```python
from build123d import *

# Parameters (mm, degrees)
F1_DEPTH = 25


with BuildPart() as f1:
    # F0 (on Right) → F1 (new body, symmetric)
    with BuildSketch(Plane.YZ):
        with BuildLine():
            Line((-68.631068, 16), (-68.631068, 0))
            Line((-68.631068, 0), (-44.032769, 0))
            Line((-44.032769, 0), (-44.032769, -22))
            Line((-44.032769, -22), (-25.631068, -22))
            ThreePointArc((-25.631068, -22), (-2.631068, 0.150878), (20.368932, -22))
            Line((20.368932, -22), (38.770634, -22))
            Line((38.770634, -22), (38.770634, 0))
            Line((38.770634, 0), (63.368932, 0))
            Line((63.368932, 0), (63.368932, 16))
            Line((63.368932, 16), (-68.631068, 16))
        make_face()
    extrude(amount=F1_DEPTH, both=True)


solid = f1.part
```
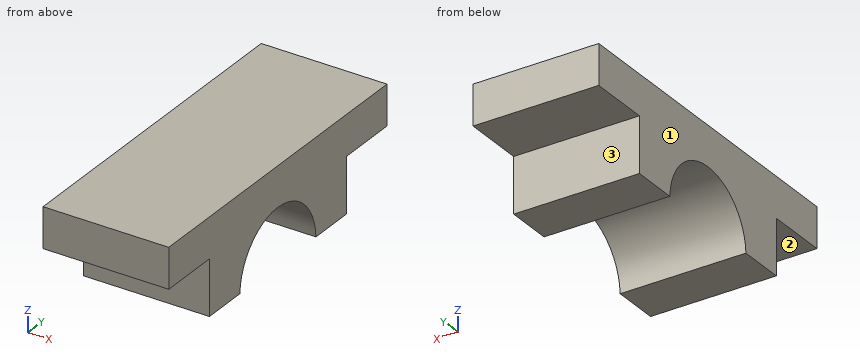
Verification items for the finished model (mm, model axes). Face numbers are marked on the shaded views. A direction names the side the tool comes from. Coordinates: 2 decimals unless noted, no trailing zeros. Loops run counter-clockwise (first coordinate to the right, second up) from the corner with the lowest first, then second, coordinate; pieces in that order, holes last. Notation, with made-up numbers: (22.25, 16) -> (28.25, 16) arc R14 ccw to (28.25, 43) -> close; hole circle Ø8 at (21.5, 43.5). An arc over 180 degrees is marked (long way). Answer in a Markdown table with one row per item. Add a question column.
1. Material ranges on probe 1 along Z at (x, y) = (-22.5, -53); probe 2 along Y at (x, z) = (10, -12.5); probe 3 along Y at (x, z) = (-8.5, -17.5), recorded low to high. Write a range as [from, to].
2. Section check C-C, the plane z = -3. Enter the section's corners in (x, y).
3. Section check D-D, the plane y = -58. Enter the section's corners in (x, z).
4. Access from +Z, -Z, +X, -X, +Y, -Y to the whole of each face (thin tool, end or side, straight path). Record for the marked faces 1, 2 and 3.
5. Depth check by flat-ended pin: P1, Ø7.5, axis at x = -12, y = -57, coming from the -Z side; P2, Ø1.5, axis at x = 19.5, y = -6, coming from the -Z side; P3, Ø3, axis at x = 15, z = -13.5, coming from the +Y side. Enter the tip coordinate at first touch or a pass-through.
6. Section check B-B, the plane x = 10. Enter the section's corners in (y, z), then the cut area to 3 significant figures.
7. Section check A-A, the plane z = -14. Enter the section's corners in (x, y).
Derived:
| question | item | result |
|---|---|---|
| 1 | probe 1 | z = [0, 16] |
| 1 | probe 2 | y = [-44.03, -23.18], [17.92, 38.77] |
| 1 | probe 3 | y = [-44.03, -25.01], [19.75, 38.77] |
| 2 | outline | (-25, -44.03) -> (25, -44.03) -> (25, -14.25) -> (-25, -14.25) -> close; (-25, 8.99) -> (25, 8.99) -> (25, 38.77) -> (-25, 38.77) -> close |
| 3 | outline | (-25, 0) -> (25, 0) -> (25, 16) -> (-25, 16) -> close |
| 4 | face 1 | +Z, -Z, -X, +Y, -Y |
| 4 | face 2 | -Z, +X, -X, -Y |
| 4 | face 3 | -Z, +X, -X, +Y |
| 5 | P1 | stops at z = 0 |
| 5 | P2 | stops at z = -0.22 |
| 5 | P3 | stops at y = 38.77 |
| 6 | outline | (-68.63, 0) -> (-44.03, 0) -> (-44.03, -22) -> (-25.63, -22) arc R23.02 cw to (20.37, -22) -> (38.77, -22) -> (38.77, 0) -> (63.37, 0) -> (63.37, 16) -> (-68.63, 16) -> close |
| 6 | area | 3,140 mm² |
| 7 | outline | (-25, -44.03) -> (25, -44.03) -> (25, -23.87) -> (-25, -23.87) -> close; (-25, 18.61) -> (25, 18.61) -> (25, 38.77) -> (-25, 38.77) -> close |
